The listing builds one solid part. Answer for the finished solid, in the listing's coordinates (mm). Face numbers are marked on the shaded views. A direction names the side the tool comes from. Coordinates: 2 decimals unless noted, no trailing zeros. Order: outer loops, then holes, each group sorted by start corner. A loop starts at its lowest first (then second) coordinate and runs counter-clockwise, first axis right, second up. Notation, with made-up numbers: (-2.5, 20.5) -> (7.5, 20.5) arc R35 ccw to (7.5, 59.5) -> close; hole circle Ø10 at (-2, 54.25). An arc over 180 degrees is marked (long way). One line per question, with ' | ' between items.
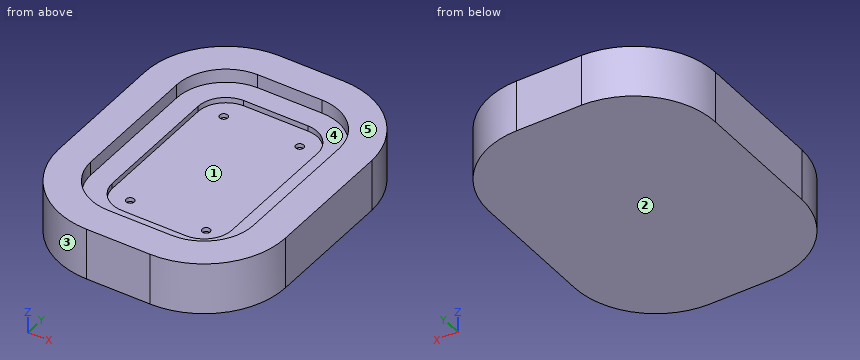
from build123d import *

# Parameters (mm, degrees)
BOSS_EXTRUDE1_START = 2.54
BOSS_EXTRUDE1_DEPTH = 24.13
BOSS_EXTRUDE2_START = -3.81
BOSS_EXTRUDE2_DEPTH = 17.78
BOSS_EXTRUDE3_START = -6.35
BOSS_EXTRUDE3_DEPTH = 15.24
SKETCH6_R           = 1.8499963
CUT_EXTRUDE1_DEPTH  = 1.905


with BuildPart() as part:
    # Sketch3 → Boss-Extrude1 (new body)
    with BuildSketch(Plane.XY.offset(BOSS_EXTRUDE1_START)):
        with BuildLine():
            Line((49.179418991, 71.83051854), (49.183589013, 10.917946581))
            ThreePointArc((49.183589013, 10.917946581), (38.030613987, -16.009405686), (11.103592243, -27.163178684))
            Line((11.103592243, -27.163178684), (-18.610242915, -27.163177904))
            ThreePointArc((-18.610242915, -27.163177904), (-45.28949294, -16.264577298), (-56.692241, 10.203124182))
            Line((-56.692241, 10.203124182), (-56.6964099, 71.109527092))
            ThreePointArc((-56.6964099, 71.109527092), (-45.79864203, 97.789054805), (-19.33135902, 109.192627907))
            Line((-19.33135902, 109.192627907), (11.095154423, 109.196819916))
            ThreePointArc((11.095154423, 109.196819916), (37.775861992, 98.2990136), (49.179418991, 71.83051854))
        make_face()
        with BuildLine():
            ThreePointArc((34.179429779, 71.6724157), (27.226556901, 87.635128483), (11.099100878, 94.196820553))
            Line((11.099100878, 94.196820553), (-19.172523946, 94.192649649))
            ThreePointArc((-19.172523946, 94.192649649), (-35.134735798, 87.239771138), (-41.696410425, 71.112801401))
            Line((-41.696410425, 71.112801401), (-41.692251788, 10.361226959))
            ThreePointArc((-41.692251788, 10.361226959), (-34.73971192, -5.601160899), (-18.612853466, -12.163178358))
            Line((-18.612853466, -12.163178358), (11.103590646, -12.163178684))
            ThreePointArc((11.103590646, -12.163178684), (27.423777198, -5.403039043), (34.183589032, 10.91728329))
            Line((34.183589032, 10.91728329), (34.179429779, 71.6724157))
        make_face(mode=Mode.SUBTRACT)
    extrude(amount=-BOSS_EXTRUDE1_DEPTH)

    # Sketch4 → Boss-Extrude2 (add)
    with BuildSketch(Plane.XY.offset(BOSS_EXTRUDE2_START)):
        with BuildLine():
            Line((-18.612853466, -12.163178358), (11.103590646, -12.163178684))
            ThreePointArc((11.103590646, -12.163178684), (27.423777198, -5.403039043), (34.183589032, 10.91728329))
            Line((34.183589032, 10.91728329), (34.179429779, 71.6724157))
            ThreePointArc((34.179429779, 71.6724157), (27.226556901, 87.635128483), (11.099100878, 94.196820553))
            Line((11.099100878, 94.196820553), (-19.172523946, 94.192649649))
            ThreePointArc((-19.172523946, 94.192649649), (-35.134735798, 87.239771138), (-41.696410425, 71.112801401))
            Line((-41.696410425, 71.112801401), (-41.692251788, 10.361226959))
            ThreePointArc((-41.692251788, 10.361226959), (-34.73971192, -5.601160899), (-18.612853466, -12.163178358))
        make_face()
        with BuildLine():
            Line((-31.696410748, 71.115398672), (-31.692261274, 10.49840121))
            ThreePointArc((-31.692261274, 10.49840121), (-27.7179266, 1.519183246), (-18.615075252, -2.163178586))
            Line((-18.615075252, -2.163178586), (11.103589581, -2.163178687))
            ThreePointArc((11.103589581, -2.163178687), (20.352576379, 1.667895757), (24.183589038, 10.916908147))
            Line((24.183589038, 10.916908147), (24.179439208, 71.535241416))
            ThreePointArc((24.179439208, 71.535241416), (20.205041728, 80.514520126), (11.102078372, 84.196820986))
            Line((11.102078372, 84.196820986), (-19.034923813, 84.1926686))
            ThreePointArc((-19.034923813, 84.1926686), (-28.014111485, 80.21827234), (-31.696410748, 71.115398672))
        make_face(mode=Mode.SUBTRACT)
    extrude(amount=-BOSS_EXTRUDE2_DEPTH)

    # Sketch5 → Boss-Extrude3 (add)
    with BuildSketch(Plane.XY.offset(BOSS_EXTRUDE3_START)):
        with BuildLine():
            Line((-18.615075252, -2.163178586), (11.103589581, -2.163178687))
            ThreePointArc((11.103589581, -2.163178687), (20.352576379, 1.667895757), (24.183589038, 10.916908147))
            Line((24.183589038, 10.916908147), (24.179439208, 71.535241416))
            ThreePointArc((24.179439208, 71.535241416), (20.205041728, 80.514520126), (11.102078372, 84.196820986))
            Line((11.102078372, 84.196820986), (-19.034923813, 84.1926686))
            ThreePointArc((-19.034923813, 84.1926686), (-28.014111485, 80.21827234), (-31.696410748, 71.115398672))
            Line((-31.696410748, 71.115398672), (-31.692261274, 10.49840121))
            ThreePointArc((-31.692261274, 10.49840121), (-27.7179266, 1.519183246), (-18.615075252, -2.163178586))
        make_face()
    extrude(amount=-BOSS_EXTRUDE3_DEPTH)

    # Sketch6 → Cut-Extrude1 (cut)
    with BuildSketch(Plane.XY.offset(-6.35)):
        with Locations((-21.53641096, 74.036821312)):
            Circle(SKETCH6_R)
        with Locations((14.02358904, 74.036821312)):
            Circle(SKETCH6_R)
        with Locations((14.02358904, 7.996821312)):
            Circle(SKETCH6_R)
        with Locations((-21.53641096, 7.996821312)):
            Circle(SKETCH6_R)
    extrude(amount=-CUT_EXTRUDE1_DEPTH, mode=Mode.SUBTRACT)


solid = part.part
Item 1: Section A-A, the plane z = -1 is taken. Give the vertices of the cut face in (x, y), plus the area to 3 significant figures.
Computed values:
outline: (-56.7, 71.11) -> (-56.69, 10.2) arc R38.08 ccw to (-18.61, -27.16) -> (11.1, -27.16) arc R38.08 ccw to (49.18, 10.92) -> (49.18, 71.83) arc R38.08 ccw to (11.1, 109.2) -> (-19.33, 109.19) arc R38.08 ccw to start; hole (-41.7, 71.11) -> (-41.69, 10.36) arc R23.08 ccw to (-18.61, -12.16) -> (11.1, -12.16) arc R23.08 ccw to (34.18, 10.92) -> (34.18, 71.67) arc R23.08 ccw to (11.1, 94.2) -> (-19.17, 94.19) arc R23.08 ccw to start | area: 5,580 mm^2
Item 2: For the marked faces 1 and 2, determine the directions among +Z, -Z, +X, -X, +Y, -Y from which every point of the face is accessible in a straight line to the end or side of a thin tool.
Computed values:
face 1: +Z | face 2: -Z, +X, -X, +Y, -Y
Item 3: Find the intervals of material crossed by L1, parallel to Y at x = 12, z = -1; L2, parallel to Y at x = -3, z = -4; L3, parallel to X at y = 64, z = -3, in increasing order.
Computed values:
L1: y = -27.15 to -12.15, 94.18 to 109.19 | L2: y = -27.16 to -2.16, 84.19 to 109.19 | L3: x = -56.7 to -41.7, 34.18 to 49.18
Item 4: Section B-B, the plane y = 89 is taken. Give the vertices of the cut face in (x, z), plus the area to 3 significant figures.
Computed values:
outline: (-52.24, -21.59) -> (44.73, -21.59) -> (44.73, 2.54) -> (25.7, 2.54) -> (25.7, -3.81) -> (-33.21, -3.81) -> (-33.21, 2.54) -> (-52.24, 2.54) -> close | area: 1,970 mm^2
Item 5: Each of these flat-tipped pins is pushed along its axis until it touches: pin 1 Ø1.1 at (x, y) = (-22, 8) entering from +Z (3 decimals); pin 2 Ø6 at (y, z) = (81, -16.5) entering from +X; pin 3 Ø1.5 at (y, z) = (-1, -6) entering from +X. Where does it stop, or does it pass through?
Computed values:
pin 1: stops at z = -8.255 | pin 2: stops at x = 48.56 | pin 3: stops at x = 47.51
Item 6: Section D-D, the plane x = -5 is taken. Give the vertices of the cut face in (y, z).
Computed values:
outline: (-27.16, -21.59) -> (109.19, -21.59) -> (109.19, 2.54) -> (94.19, 2.54) -> (94.19, -3.81) -> (84.19, -3.81) -> (84.19, -6.35) -> (-2.16, -6.35) -> (-2.16, -3.81) -> (-12.16, -3.81) -> (-12.16, 2.54) -> (-27.16, 2.54) -> close
Item 7: Section C-C, the plane z = -13.25 is taken. Give the vertices of the cut face in (x, y), plus the area to 3 significant figures.
Computed values:
outline: (-56.7, 71.11) -> (-56.69, 10.2) arc R38.08 ccw to (-18.61, -27.16) -> (11.1, -27.16) arc R38.08 ccw to (49.18, 10.92) -> (49.18, 71.83) arc R38.08 ccw to (11.1, 109.2) -> (-19.33, 109.19) arc R38.08 ccw to start | area: 13,200 mm^2
Item 8: Determine the mould class of the marked faces 3, 4 and 5 for opening direction Y: pulls with the +Y half, pulls with the -Y half, needs draft (parallel to the pull), parting line crosses it, or undercut.
Computed values:
face 3: pulls with the -Y half | face 4: undercut | face 5: needs draft
